Work out the finished part from the listing and answer in its coordinate system (mm). A direction names the side the tool comes from. Round coordinates to 2 decimals unless told otherwise and drop trailing zeros. Write each loop counter-clockwise with the first axis right and the second up, starting at its lowest first coordinate (ties: lowest second). Pieces come first, ordered by that corner, then holes. Notation, with made-up numbers: (19.25, 27) -> (39.25, 27) arc R8 ccw to (39.25, 36) -> close; hole circle Ø10 at (-39, 20.5). An arc over 180 degrees is marked (long way). One line per item, written item: value.
```python
from build123d import *

# Parameters (mm, degrees)
F0_W      = 101.6
F0_H      = 76.2
F0_R      = 3.175
F1_DEPTH  = 203.2
F2_R      = 25.4
F3_DEPTH  = 101.6
F4_R      = 31.75
F5_DEPTH  = 190.5
F6_R      = 12.69999
F7_R      = 3.175
F7_R_2    = 35.56
F8_DEPTH  = 127
F10_W     = 101.6
F10_H     = 76.2
F11_DEPTH = 5.08


# Not quite as in the source:
# - a fillet or chamfer is up to 0.001 mm smaller than in the source, because OpenCascade refuses the exact size


with BuildPart() as f1:
    # F0 (on Top) → F1 (new body)
    with BuildSketch(Plane.XY):
        Rectangle(F0_W, F0_H)
        with Locations((-45.085, -28.5786420731)):
            Circle(F0_R, mode=Mode.SUBTRACT)
        with Locations((45.085, -28.5786420731)):
            Circle(F0_R, mode=Mode.SUBTRACT)
        with Locations((-45.085, 29.3072120343)):
            Circle(F0_R, mode=Mode.SUBTRACT)
        with Locations((45.085, 29.3072120343)):
            Circle(F0_R, mode=Mode.SUBTRACT)
    extrude(amount=F1_DEPTH)

    # F2 (on face) → F3 (cut)
    with BuildSketch(Plane.YZ.offset(50.8)):
        with Locations((0, 38.1)):
            Circle(F2_R)
    extrude(amount=-F3_DEPTH, mode=Mode.SUBTRACT)

    # F4 (on face) → F5 (cut)
    with BuildSketch(Plane.XY.offset(203.2)):
        Circle(F4_R)
    extrude(amount=-F5_DEPTH, mode=Mode.SUBTRACT)

    # F6 (radius 12.7 in the source; OpenCascade refuses exactly that, so slightly less here)
    f6_edges = [f1.edges().sort_by_distance(p)[0] for p in [
        (-50.8, 38.1, 101.6),
        (-50.8, -38.1, 101.6),
        (50.8, -38.1, 101.6),
        (50.8, 38.1, 101.6),
    ]]
    fillet(f6_edges, radius=F6_R)

    # F7 (on face) → F8 (cut)
    with BuildSketch(Plane.XY.offset(203.2)):
        with BuildLine():
            ThreePointArc((50.8, 25.40001), (47.08025905, 34.38025905), (38.10001, 38.1))
            Line((38.10001, 38.1), (-38.10001, 38.1))
            ThreePointArc((-38.10001, 38.1), (-47.08025905, 34.38025905), (-50.8, 25.40001))
            Line((-50.8, 25.40001), (-50.8, -25.40001))
            ThreePointArc((-50.8, -25.40001), (-47.08025905, -34.38025905), (-38.10001, -38.1))
            Line((-38.10001, -38.1), (38.10001, -38.1))
            ThreePointArc((38.10001, -38.1), (47.08025905, -34.38025905), (50.8, -25.40001))
            Line((50.8, -25.40001), (50.8, 25.40001))
        make_face()
        with Locations((-45.085, -28.5786420731)):
            Circle(F7_R, mode=Mode.SUBTRACT)
        with Locations((45.085, -28.5786420731)):
            Circle(F7_R, mode=Mode.SUBTRACT)
        Circle(F7_R_2, mode=Mode.SUBTRACT)
        with Locations((-45.085, 29.3072120343)):
            Circle(F7_R, mode=Mode.SUBTRACT)
        with Locations((45.085, 29.3072120343)):
            Circle(F7_R, mode=Mode.SUBTRACT)
    extrude(amount=-F8_DEPTH, mode=Mode.SUBTRACT)

    # F10 (on offset) → F11 (join)
    with BuildSketch(Plane.XY.offset(203.2)):
        Rectangle(F10_W, F10_H)
    extrude(amount=F11_DEPTH)


solid = f1.part
```
(1) Find section D-D on z = 69. Give the vertices of the cut face in (x, y) (3 decimals).
Reported:
outline: (-50.8, -25.4) arc R12.7 ccw to (-38.1, -38.1) -> (38.1, -38.1) arc R12.7 ccw to (50.8, -25.4) -> (50.8, 25.4) arc R12.7 ccw to (38.1, 38.1) -> (-38.1, 38.1) arc R12.7 ccw to (-50.8, 25.4) -> close; hole circle Ø6.35 at (-45.085, -28.579); hole circle Ø6.35 at (-45.085, 29.307); hole circle Ø63.5 at (0, 0); hole circle Ø6.35 at (45.085, -28.579); hole circle Ø6.35 at (45.085, 29.307)
(2) A tool of negligible diameter and unlimited length cuts with its end or side. For faces 3 (the face through (0, 0, 12.7)), 4 (the face through (-45.77, -31.68, 37.57)), 5 (the face through (50.8, 0, 12)), from which of +Z, -Z, +X, -X, +Y, -Y can it reach the whole face along a straight path? Write none if from no direction.
Reported:
face 3: none
face 4: -Z
face 5: +Z, -Z, +X, +Y, -Y
(3) For a pull along Z with two mould halves and no side action, classify faces 1 (the face through (46.98, 34.48, 38.63)), 2 (the face through (0, 0, 203.2)) as pulls with the +Z half, pulls with the -Z half, needs draft (parallel to the pull), parting line crosses it, or undercut.
Reported:
face 1: needs draft
face 2: undercut
(4) Flat-ended cylindrical pins translate along their axes: pin 1 Ø5 at (x, z) = (11, 105.5) entering from -Y; pin 2 Ø4 at (y, z) = (24.5, 115) entering from +X; pin 3 Ø3 at (x, z) = (31, 181) entering from -Y. Find the tip coordinate at first contact, or state that the pin passes through.
Reported:
pin 1: stops at y = -34.53
pin 2: stops at x = 27.54
pin 3: stops at y = -19.86
(5) Find section B-B on y = -15.5. Give the vertices of the cut face in (x, z), plus the area to 3 significant figures.
Reported:
outline: (-50.8, 0) -> (50.8, 0) -> (50.8, 17.98) -> (27.71, 17.98) -> (27.71, 12.7) -> (-27.71, 12.7) -> (-27.71, 17.98) -> (-50.8, 17.98) -> close; (-50.8, 58.22) -> (-27.71, 58.22) -> (-27.71, 203.2) -> (27.71, 203.2) -> (27.71, 58.22) -> (50.8, 58.22) -> (50.8, 76.2) -> (32, 76.2) -> (32, 203.2) -> (50.8, 203.2) -> (50.8, 208.28) -> (-50.8, 208.28) -> (-50.8, 203.2) -> (-32, 203.2) -> (-32, 76.2) -> (-50.8, 76.2) -> close
area: 3,970 mm2
(6) Find section A-A on z = 38.1. Give the number of separate pieces and of enclosed holes in the cut face, plus the area to 3 significant figures.
Reported:
separate pieces: 2
enclosed holes: 4
area: 1,990 mm2
(7) Consider probe 1 along Z at (x, y) = (9.5, -18.5); probe 2 along X at (y, z) = (1.5, 142); probe 3 along Z at (x, y) = (-45.5, -11.5). Determine where each line is inside the solid, lowest interval first.
Reported:
probe 1: z = 0 to 12.7, 203.2 to 208.28
probe 2: x = -35.53 to -31.71, 31.71 to 35.53
probe 3: z = 0 to 15.45, 60.75 to 76.2, 203.2 to 208.28
(8) Find section C-C on x = -9. Give the vertices of the cut face in (y, z).
Reported:
outline: (-38.1, 0) -> (38.1, 0) -> (38.1, 76.2) -> (34.4, 76.2) -> (34.4, 203.2) -> (38.1, 203.2) -> (38.1, 208.28) -> (-38.1, 208.28) -> (-38.1, 203.2) -> (-34.4, 203.2) -> (-34.4, 76.2) -> (-38.1, 76.2) -> close; hole (-30.45, 12.7) -> (30.45, 12.7) -> (30.45, 203.2) -> (-30.45, 203.2) -> close
